```python
from build123d import *

# Parameters (mm, degrees)
SKETCH3_R           = 290
SKETCH3_R_2         = 240
BOSS_EXTRUDE1_DEPTH = 60
FILLET1_R           = 24
SHELL1_T            = -3


with BuildPart() as part:
    # Sketch3 → Boss-Extrude1 (new body)
    with BuildSketch(Plane(origin=(0, 0, 0), x_dir=(0, 0, -1), z_dir=(1, 0, 0))):
        Circle(SKETCH3_R)
        Circle(SKETCH3_R_2, mode=Mode.SUBTRACT)
    extrude(amount=BOSS_EXTRUDE1_DEPTH)

    # Fillet1
    fillet1_edges = [part.edges().sort_by_distance(p)[0] for p in [
        (0, 0, 290),
        (60, 0, 290),
    ]]
    fillet(fillet1_edges, radius=FILLET1_R)

    # Shell1
    shell1_openings = [part.faces().sort_by_distance(p)[0] for p in [
        (30, 0, 240),
    ]]
    offset(amount=SHELL1_T, openings=shell1_openings, kind=Kind.INTERSECTION)


solid = part.part
```
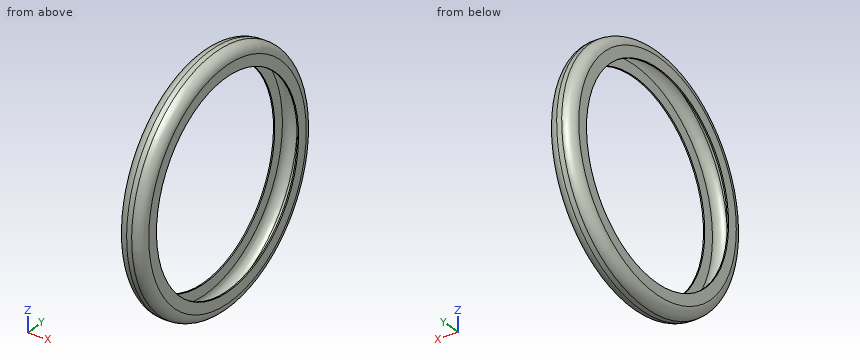
Could you check a few things on this model? Use its own coordinates, in mm. Round coordinates to 2 decimals unless told otherwise and drop trailing zeros. Order: outer loops, then holes, each group sorted by start corner. A loop starts at its lowest first (then second) coordinate and runs counter-clockwise, first axis right, second up. Notation, with made-up numbers: (31.25, 1) -> (73.25, 1) arc R15 cw to (73.25, 9) -> close; hole circle Ø8 at (79, -28). An arc over 180 degrees is marked (long way). One line per question, with ' | ' between items.
Q1. If we section it at C-C on x = 16.5: Write out the boundary of the cut face in (y, z).
Computed values:
outline: circle Ø577.6 at (0, 0); hole circle Ø571.23 at (0, 0)
Q2. If I drill on line 1 (X direction, y = -2, z = 246.5); line 2 (Y direction, x = 27, z = 0); line 3 (X direction, y = -49, z = -264), over which ranges is the centre line in solid material (lowest first)? Write a range as from..to.
Computed values:
line 1: 0..3, 57..60 | line 2: -290..-287, 287..290 | line 3: 0.13..3.15, 56.85..59.87
Q3. I'm going to push flat-ended pins straight in: pin 1 (2 mm diameter, centred on x = 39.5, z = -29, fed in from -Y); pin 2 (3 mm diameter, centred on x = 44.5, y = 30.5, fed in from -Z); pin 3 (2 mm diameter, centred on x = 21.5, z = -44.5, fed in from +Y). Where does each tip first touch, or does it pass through?
Computed values:
pin 1: y = -288.45 | pin 2: z = -287.37 | pin 3: y = 286.61
Q4. If we section it at A-A on z = 0: Write out the boundary of the cut face in (x, y).
Computed values:
outline: (0, -266) arc R24 ccw to (24, -290) -> (36, -290) arc R24 ccw to (60, -266) -> (60, -240) -> (57, -240) -> (57, -266) arc R21 cw to (36, -287) -> (24, -287) arc R21 cw to (3, -266) -> (3, -240) -> (0, -240) -> close; (0, 240) -> (3, 240) -> (3, 266) arc R21 cw to (24, 287) -> (36, 287) arc R21 cw to (57, 266) -> (57, 240) -> (60, 240) -> (60, 266) arc R24 ccw to (36, 290) -> (24, 290) arc R24 ccw to (0, 266) -> close
Q5. If we section it at D-D on x = 45.5: Write out the boundary of the cut face in (y, z).
Computed values:
outline: circle Ø576.08 at (0, 0); hole circle Ø569.46 at (0, 0)
